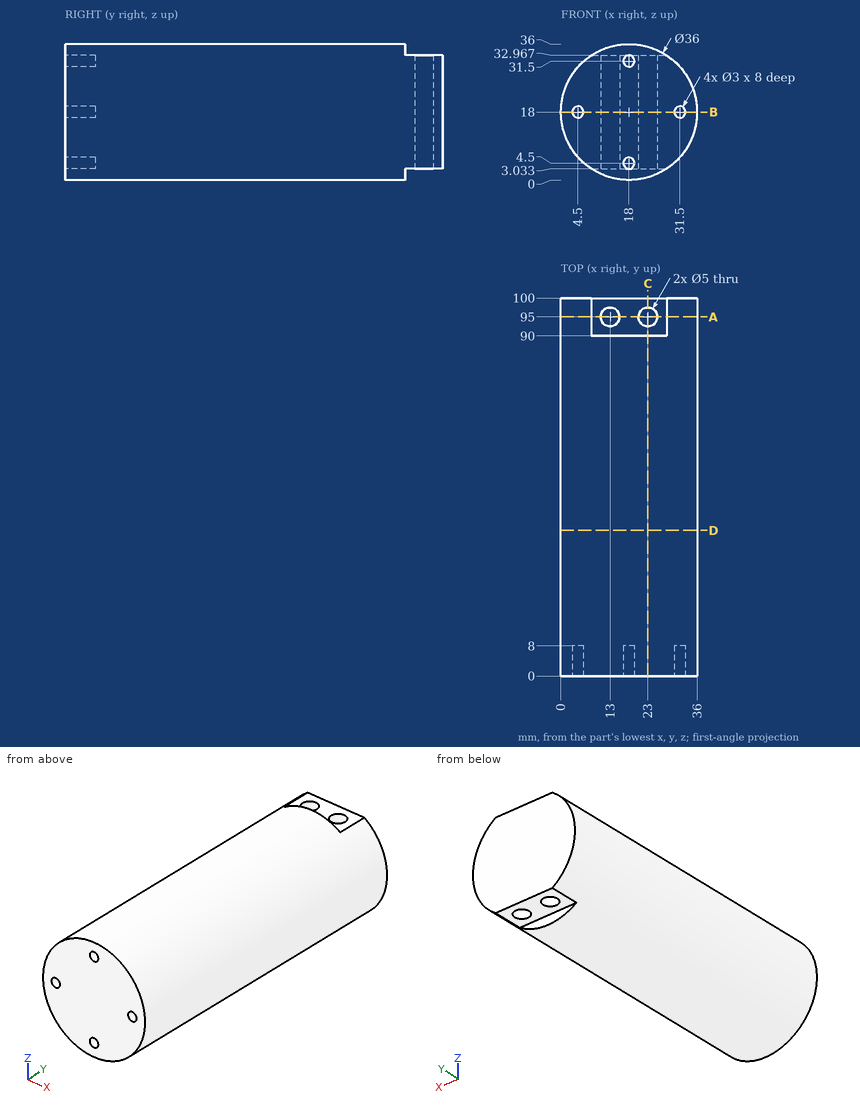
Can you work these out from the drawing? Everything is in mm from the part's minimum corner. Give positions to 0.01 mm unless a question says otherwise; leave off trailing zeros. Loops run counter-clockwise (first coordinate to the right, second up) from the corner with the lowest first, then second, coordinate; pieces in that order, holes last. Notation, with made-up numbers: (43, 67) -> (57, 67) arc R11 ccw to (57, 71) -> close; hole circle Ø10 at (22, -19.5). An arc over 180 degrees is marked (long way). Return JSON: item names as keys, results as strings.
Q1. I want a section at A-A, the plane y = 95. List the corners of the cut face in (x, z) for me, then the cut area to 3 significant figures.
Checks:
{"outline": "(8, 3.03) -> (10.5, 3.03) -> (10.5, 32.97) -> (8, 32.97) arc R18 ccw to start; (15.5, 3.03) -> (20.5, 3.03) -> (20.5, 32.97) -> (15.5, 32.97) -> close; (25.5, 3.03) -> (28, 3.03) arc R18 ccw to (28, 32.97) -> (25.5, 32.97) -> close", "area": "636 mm2"}
Q2. I need wall thicknesses on probe 1 along Z at (x, y) = (18, 5); probe 2 along Y at (x, z) = (23, 21.5); probe 3 along X at (y, z) = (69.5, 8) (1 decimal). Which ranges of each line are inside material? Lowest first, please.
Checks:
{"probe 1": "z = 0 to 3, 6 to 30, 33 to 36", "probe 2": "y = 0 to 92.5, 97.5 to 100", "probe 3": "x = 3 to 33"}
Q3. I want a section at C-C, the plane x = 23. List the corners of the cut face in (y, z) for me, then the cut area to 3 significant figures.
Checks:
{"outline": "(0, 0.71) -> (90, 0.71) -> (90, 3.03) -> (92.5, 3.03) -> (92.5, 32.97) -> (90, 32.97) -> (90, 35.29) -> (0, 35.29) -> close; (97.5, 3.03) -> (100, 3.03) -> (100, 32.97) -> (97.5, 32.97) -> close", "area": "3,260 mm2"}
Q4. For pin 1 Ø10 at (y, z) = (47.5, 8) entering from +X; pin 2 Ø2.5 at (x, z) = (18, 31.5) entering from -Y; pin 3 Ø0.9 at (x, z) = (18.5, 2) entering from +Y; pin 4 Ø4 at (x, y) = (13, 95) entering from +Z, each with a flat end and sliding along its axis, tell me the tip position at first contact or that it passes through.
Checks:
{"pin 1": "stops at x = 35.29", "pin 2": "stops at y = 8", "pin 3": "stops at y = 90", "pin 4": "passes through"}
Q5. I want a section at B-B, the plane z = 18. List the corners of the cut face in (x, y) for me, then the cut area to 3 significant figures.
Checks:
{"outline": "(0, 0) -> (3, 0) -> (3, 8) -> (6, 8) -> (6, 0) -> (30, 0) -> (30, 8) -> (33, 8) -> (33, 0) -> (36, 0) -> (36, 100) -> (0, 100) -> close; hole circle Ø5 at (13, 95); hole circle Ø5 at (23, 95)", "area": "3,510 mm2"}
Q6. I want a section at D-D, the plane y = 38.5. List the corners of the cut face in (x, z) for me, then the cut area to 3 significant figures.
Checks:
{"outline": "circle Ø36 at (18, 18)", "area": "1,020 mm2"}
